The listing builds one solid part. Answer for the finished solid, in the listing's coordinates (mm). A direction names the side the tool comes from. Give positions to 0.01 mm unless a question says otherwise; leave off trailing zeros. Write each loop counter-clockwise with the first axis right and the second up, starting at its lowest first coordinate (ties: lowest second). Pieces come first, ordered by that corner, then holes.
```python
from build123d import *

# Parameters (mm, degrees)
F0_W     = 304.8
F0_H     = 12.7
F1_DEPTH = 101.6
F2_R     = 19.05
F2_R_2   = 13.335
F3_DEPTH = 152.4
F4_R     = 5.55625
F5_DEPTH = 25.4
F6_R     = 31.75
F6_R_2   = 25.4
F7_DEPTH = 76.2


with BuildPart() as f1:
    # F0 (on Front) → F1 (new body, symmetric)
    with BuildSketch(Plane.XZ):
        Rectangle(F0_W, F0_H)
    extrude(amount=F1_DEPTH, both=True)

    # F2 (on face) → F3 (join)
    with BuildSketch(Plane(origin=(0, 0, -6.35), x_dir=(1, 0, 0), z_dir=(0, 0, -1))):
        with Locations((101.6, 0)):
            Circle(F2_R)
        with Locations((101.6, 0)):
            Circle(F2_R_2, mode=Mode.SUBTRACT)
        with Locations((-101.6, 0)):
            Circle(F2_R)
        with Locations((-101.6, 0)):
            Circle(F2_R_2, mode=Mode.SUBTRACT)
    extrude(amount=F3_DEPTH)

    # F4 (on face) → F5 (cut)
    with BuildSketch(Plane.XY.offset(6.35)):
        Circle(F4_R)
    extrude(amount=-F5_DEPTH, mode=Mode.SUBTRACT)

    # F6 (on face) → F7 (join)
    with BuildSketch(Plane.XY.offset(6.35)):
        Circle(F6_R)
        Circle(F6_R_2, mode=Mode.SUBTRACT)
    extrude(amount=F7_DEPTH)


solid = f1.part
```
Item 1: Determine the mould class of faces 1 (the face through (-98, -13, -158.75)), 2 (the face through (-5.506, -24.796, 43.917)), 3 (the face through (152.4, -1, 0)) for opening direction X: pulls with the +X half, pulls with the -X half, needs draft (parallel to the pull), parting line crosses it, or undercut.
Conclusion:
face 1: needs draft
face 2: undercut
face 3: pulls with the +X half
Item 2: Each of these flat-tipped pins is pushed along its axis until it touches: P1, Ø6.5, axis at x = 0, y = 0, coming from the -Z side; P2, Ø8, axis at x = 96, y = 33.5, coming from the -Z side; P3, Ø1, axis at y = 12.5, z = 54, coming from the -X side; P4, Ø1, axis at y = -13, z = 31.5, coming from the -X side. Where does it stop, or does it pass through?
Conclusion:
P1: passes through
P2: stops at z = -6.35
P3: stops at x = -29.39
P4: stops at x = -29.19
Item 3: Which of the six approach directions +Z, -Z, +X, -X, +Y, -Y give full straight-line access (tool end or side, diameter ignored) to faces 4 (the face through (119.197, 7.296, -81.483)), 5 (the face through (0, -6, 6.35)), 6 (the face through (-2, 101.6, 0))?
Conclusion:
face 4: -Z
face 5: +Z
face 6: +Z, -Z, +X, -X, +Y
Item 4: A cutting plane is placed at C-C, the plane z = -97. Give the vertices of the cut face in (x, y) (3 decimals), plus the area to 3 significant figures.
Conclusion:
outline: circle Ø38.1 at (-101.6, 0); circle Ø38.1 at (101.6, 0); hole circle Ø26.67 at (-101.6, 0); hole circle Ø26.67 at (101.6, 0)
area: 1,160 mm2
Item 5: Consider probe 1 along X at (y, z) = (0, -92) (3 decimals); probe 2 along Y at (x, z) = (0, 56.5); probe 3 along Y at (x, z) = (-101, -69). Determine where each line is inside the solid, lowest interval first.
Conclusion:
probe 1: x = -120.65 to -114.935, -88.265 to -82.55, 82.55 to 88.265, 114.935 to 120.65
probe 2: y = -31.75 to -25.4, 25.4 to 31.75
probe 3: y = -19.04 to -13.32, 13.32 to 19.04
Item 6: A cutting plane is placed at B-B, the plane x = 0. Give the vertices of the cut face in (y, z).
Conclusion:
outline: (-101.6, -6.35) - (-5.56, -6.35) - (-5.56, 6.35) - (-25.4, 6.35) - (-25.4, 82.55) - (-31.75, 82.55) - (-31.75, 6.35) - (-101.6, 6.35) - close; (5.56, -6.35) - (101.6, -6.35) - (101.6, 6.35) - (31.75, 6.35) - (31.75, 82.55) - (25.4, 82.55) - (25.4, 6.35) - (5.56, 6.35) - close
Item 7: A cutting plane is placed at D-D, the plane z = 62. Give the vertices of the cut face in (x, y), plus the area to 3 significant figures.
Conclusion:
outline: circle Ø63.5 at (0, 0); hole circle Ø50.8 at (0, 0)
area: 1,140 mm2
